```python
from build123d import *

# Parameters (mm, degrees)
SKETCH_W     = 12
SKETCH_H     = 12
SKETCH001_R  = 4
SKETCH002_R  = 3.1
POCKET_DEPTH = 10.001


with BuildPart() as part:
    # Sketch → AdditiveLoft section 0
    with BuildSketch(Plane.XY):
        Rectangle(SKETCH_W, SKETCH_H)
    # Sketch001 (on DatumPlane) → AdditiveLoft section 1
    with BuildSketch(Plane.XY.offset(10)):
        Circle(SKETCH001_R)
    loft()

    # Sketch002 (on DatumPlane) → Pocket (cut, through all)
    with BuildSketch(Plane.XY.offset(10)):
        Circle(SKETCH002_R)
    extrude(amount=-POCKET_DEPTH, mode=Mode.SUBTRACT)


solid = part.part
```
Part model, mm, in its own coordinate system. Coordinates: 2 decimals unless noted, no trailing zeros. Return JSON: item names as keys, results as strings. Group by question number.
Item 1: Pull direction X, two halves, no side cores. Call faces 1 (the face through (2, -3, 10)), 2 (the face through (1.43, -2.75, 5.07)): pulls with the +X half, pulls with the -X half, needs draft (parallel to the pull), parting line crosses it, or undercut.
Item 2: Drill centre lines: probe 1 along X at (y, z) = (-0.5, 3); probe 2 along X at (y, z) = (-1.5, 8.5); probe 3 along Y at (x, z) = (0, 3). Where is each one in solid material? Low to high. Write a range as from..to.
Item 3: Pin check, flat tips, straight feed: pin 1 (5 mm diameter, centred on x = -0.5, z = 6, fed in from -Y); pin 2 (5 mm diameter, centred on x = 0, y = 0, fed in from +Z); pin 3 (1 mm diameter, centred on x = 3, z = 8, fed in from +Y); pin 4 (1.5 mm diameter, centred on x = -2.5, z = 3.5, fed in from +Y). Stop position of each tip, or through.
Check values:
{
 "1": {"face 1": "needs draft", "face 2": "undercut"},
 "2": {"probe 1": "x = -5.4..-3.06, 3.06..5.4", "probe 2": "x = -4.11..-2.71, 2.71..4.11", "probe 3": "y = -5.4..-3.1, 3.1..5.4"},
 "3": {"pin 1": "stops at y = -5.3", "pin 2": "passes through", "pin 3": "stops at y = 4", "pin 4": "stops at y = 5.38"}
}
